For this review, take the finished solid that the model builds, in its own axes (mm). Face numbers are marked on the shaded views. Coordinates: 2 decimals unless noted, no trailing zeros. Write each loop counter-clockwise with the first axis right and the second up, starting at its lowest first coordinate (ties: lowest second). Pieces come first, ordered by that corner, then holes. Notation, with made-up numbers: (-5, 71.5) - (14, 71.5) arc R33 ccw to (14, 102.5) - close; hole circle Ø10 at (-28, 44.25). An arc over 180 degrees is marked (long way). Use one line per item in the form item = value. Start each with the question number.
1) We need section C-C (z = -37). Give the boundary of the cut face in (x, y), plus the area to 3 significant figures.
2) We need section B-B (x = 459.5). Give the boundary of the cut face in (y, z) (3 decimals).
3) For L1, parallel to Y at x = 254, z = 14.5; L2, parallel to X at y = 916, z = 32.5; L3, parallel to Y at x = 186, z = 33, list the stretches that pass through material, from the lowest coordinate up. Write a range as from..to.
4) Mouldability with a two-part tool opening along Y and no side actions: class the marked faces 1 and 2 as pulls with the +Y half, pulls with the -Y half, needs draft (parallel to the pull), parting line crosses it, or undercut.
5) Insertion check: P1, Ø5, axis at x = 365.5, y = 873, coming from the +Z side; P2, Ø3, axis at y = 382.5, z = -6.5, coming from the +X side; P3, Ø4, axis at y = 625, z = -32, coming from the -X side. Each pin has a flat end and moves straight along its axis. Give the tip position at first contact, or say it passes through.
6) We need section A-A (y = 704). Give the boundary of the cut face in (x, z) (3 decimals), plus the area to 3 significant figures.
7) We need section D-D (x = 133). Give the boundary of the cut face in (y, z) (3 decimals).
```python
from build123d import *

# Parameters (mm, degrees)
F0_W     = 596.9
F0_H     = 1099.82
F0_W_2   = 558.8
F0_H_2   = 1061.72
F1_DEPTH = 38.1
F2_W     = 1099.82
F2_H     = 9.525
F3_DEPTH = 584.2
F4_W     = 558.8
F4_H     = 1061.72
F5_DEPTH = 19.05
F6_W     = 482.6
F6_H     = 38.1
F6_H_2   = 782.32
F7_DEPTH = 88.9


with BuildPart() as f1:
    # F0 (on Top) → F1 (new body)
    with BuildSketch(Plane.XY):
        with Locations((199.572543, 475.369852)):
            Rectangle(F0_W, F0_H)
        with Locations((199.572543, 475.369852)):
            Rectangle(F0_W_2, F0_H_2, mode=Mode.SUBTRACT)
    extrude(amount=F1_DEPTH)

    # F2 (on face) → F3 (join)
    with BuildSketch(Plane(origin=(-98.877457, 0, 0), x_dir=(0, -1, 0), z_dir=(-1, 0, 0))):
        with Locations((-475.369852, 26.9875)):
            Rectangle(F2_W, F2_H)
    extrude(amount=-F3_DEPTH)

    # F4 (on face) → F5 (join)
    with BuildSketch(Plane(origin=(0, 0, 22.225), x_dir=(1, 0, 0), z_dir=(0, 0, -1))):
        with Locations((199.572543, -475.369852)):
            Rectangle(F4_W, F4_H)
        Polygon((440.872543, -968.129852), (-41.727457, -968.129852), (-41.727457, -904.629852), (-41.727457, -866.529852), (-41.727457, -84.209852), (-41.727457, -46.109852), (-41.727457, 17.390148), (440.872543, 17.390148), (440.872543, -46.109852), (440.872543, -84.209852), (440.872543, -866.529852), (440.872543, -904.629852), align=None, mode=Mode.SUBTRACT)
    extrude(amount=F5_DEPTH)

    # F6 (on face) → F7 (join)
    with BuildSketch(Plane(origin=(0, 0, 22.225), x_dir=(1, 0, 0), z_dir=(0, 0, -1))):
        with Locations((199.572543, -885.579852)):
            Rectangle(F6_W, F6_H)
        with Locations((199.572543, -65.159852)):
            Rectangle(F6_W, F6_H)
        with Locations((199.572543, -475.369852)):
            Rectangle(F6_W, F6_H_2)
    extrude(amount=F7_DEPTH)


solid = f1.part
```
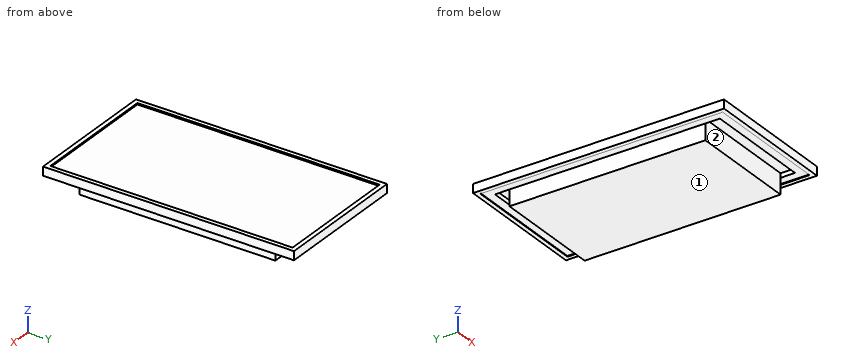
Determined:
q1.outline = (-41.73, 46.11) - (440.87, 46.11) - (440.87, 904.63) - (-41.73, 904.63) - close
q1.area = 414,000 mm²
q2.outline = (-74.54, 0) - (-55.49, 0) - (-55.49, 3.175) - (1006.23, 3.175) - (1006.23, 0) - (1025.28, 0) - (1025.28, 38.1) - (1006.23, 38.1) - (1006.23, 31.75) - (-55.49, 31.75) - (-55.49, 38.1) - (-74.54, 38.1) - close
q3.L1 = -74.54..-17.39, 46.11..904.63, 968.13..1025.28
q3.L2 = -98.88..-79.83, 478.97..498.02
q3.L3 = -74.54..-55.49, 1006.23..1025.28
q4.face_1 = needs draft
q4.face_2 = undercut
q5.P1 = 31.75
q5.P2 = 440.87
q5.P3 = -41.73
q6.outline = (-98.877, 0) - (-79.827, 0) - (-79.827, 3.175) - (-41.727, 3.175) - (-41.727, -66.675) - (440.873, -66.675) - (440.873, 3.175) - (478.973, 3.175) - (478.973, 0) - (498.023, 0) - (498.023, 38.1) - (478.973, 38.1) - (478.973, 31.75) - (-79.827, 31.75) - (-79.827, 38.1) - (-98.877, 38.1) - close
q6.area = 51,100 mm²
q7.outline = (-74.54, 0) - (-55.49, 0) - (-55.49, 3.175) - (-17.39, 3.175) - (-17.39, 22.225) - (46.11, 22.225) - (46.11, -66.675) - (904.63, -66.675) - (904.63, 22.225) - (968.13, 22.225) - (968.13, 3.175) - (1006.23, 3.175) - (1006.23, 0) - (1025.28, 0) - (1025.28, 38.1) - (1006.23, 38.1) - (1006.23, 31.75) - (-55.49, 31.75) - (-55.49, 38.1) - (-74.54, 38.1) - close
